Design review of the part built by this model. Coordinates are the model's own, in mm. Face numbers are marked on the shaded views. A direction names the side the tool comes from. Give positions to 0.01 mm unless a question says otherwise; leave off trailing zeros. Write each question's results on one line, items separated by ' | '. Start each with the question number.
from build123d import *

# Parameters (mm, degrees)
F1_DEPTH = 2
F2_R     = 0.99999


# Not quite as in the source:
# - a fillet or chamfer is up to 0.001 mm smaller than in the source, because OpenCascade refuses the exact size


with BuildPart() as f1:
    # F0 (on Top) → F1 (new body)
    with BuildSketch(Plane.XY):
        with BuildLine():
            ThreePointArc((-13.75, 3.75), (-14.4571067812, 3.4571067812), (-14.75, 2.75))
            Line((-14.75, 2.75), (-14.75, -2.75))
            ThreePointArc((-14.75, -2.75), (-14.4571067812, -3.4571067812), (-13.75, -3.75))
            Line((-13.75, -3.75), (13.75, -3.75))
            ThreePointArc((13.75, -3.75), (14.4571067812, -3.4571067812), (14.75, -2.75))
            Line((14.75, -2.75), (14.75, 2.75))
            ThreePointArc((14.75, 2.75), (14.4571067812, 3.4571067812), (13.75, 3.75))
            Line((13.75, 3.75), (-13.75, 3.75))
        make_face()
        with BuildLine():
            Line((-11.75, 1.75), (11.75, 1.75))
            ThreePointArc((11.75, 1.75), (12.4571067812, 1.4571067812), (12.75, 0.75))
            Line((12.75, 0.75), (12.75, -0.75))
            ThreePointArc((12.75, -0.75), (12.4571067812, -1.4571067812), (11.75, -1.75))
            Line((11.75, -1.75), (-11.75, -1.75))
            ThreePointArc((-11.75, -1.75), (-12.4571067812, -1.4571067812), (-12.75, -0.75))
            Line((-12.75, -0.75), (-12.75, 0.75))
            ThreePointArc((-12.75, 0.75), (-12.4571067812, 1.4571067812), (-11.75, 1.75))
        make_face(mode=Mode.SUBTRACT)
    extrude(amount=F1_DEPTH)

    # F2 (radius 1 in the source; OpenCascade refuses exactly that, so slightly less here)
    f2_edges = [f1.edges().sort_by_distance(p)[0] for p in [
        (0, 1.75, 2),
        (0, 1.75, 0),
        (0, 3.75, 0),
        (0, -3.75, 2),
    ]]
    fillet(f2_edges, radius=F2_R)


solid = f1.part
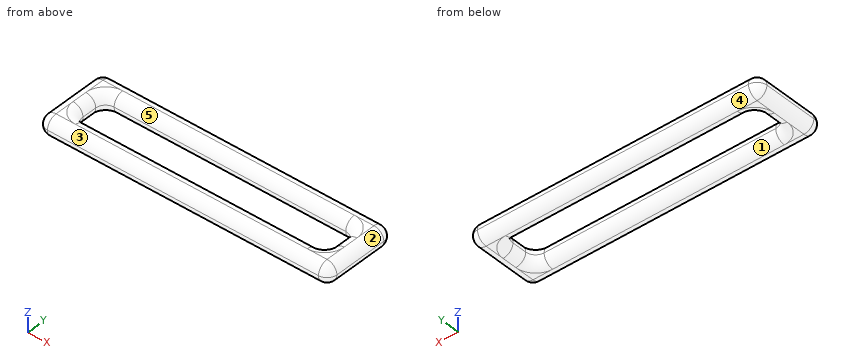
Q1. Insertion check: P1, Ø1, axis at y = 2.5, z = 0.5, coming from the -X side. The pin has a flat end and moves straight along its axis. Give the tip position at first contact, or say it passes through.
Q2. Machinability: for the marked faces 1 and 2, which of the approach directions +Z, -Z, +X, -X, +Y, -Y give a long, thin tool a straight path to every point of the face, cutting with its end or side? Answer none if there is none.
Q3. The part is to be moulded in two halves that separate along Y. For the marked faces 3, 4 and 5, say which applies: +Y half, -Y half, draft (parallel to the pull), parting line (faces both ways), or undercut.
Q4. For line 1 along Y through (x, z) = (-3.75, 0.95); line 2 along X through (y, z) = (1.75, 0.35); line 3 along Y through (x, z) = (13, 0.95), list the stretches that pass through material, from the lowest coordinate up. Write a range as [from, to].
Result:
1) P1: stops at x = -14.75
2) face 1: -Z | face 2: +Z, +X, +Y, -Y
3) face 3: -Y half | face 4: +Y half | face 5: undercut
4) line 1: y = [-3.75, -1.75], [1.75, 3.75] | line 2: x = [-14.51, -12.48], [12.48, 14.51] | line 3: y = [-3.75, 3.75]
